Autodesk Inventor part; units mm, degrees
ref_plane "YZ Plane" through (0, 0, 0) normal (1, 0, 0) x (0, 1, 0)
ref_plane "XZ Plane" through (0, 0, 0) normal (0, 1, 0) x (-1, 0, 0)
ref_plane "XY Plane" through (0, 0, 0) normal (0, 0, 1) x (1, 0, 0)
sketch "Skizze1" plane through (0, 0, 0) normal (0, 0, 1) x (1, 0, 0)
  line L0 (0, 0) -> (100, 0)
  line L1 (100, 0) -> (100, 60)
  line L2 (100, 60) -> (0, 60)
  line L3 (0, 60) -> (0, 0)
  dimension "d0" = 100
  dimension "d1" = 60
extrude "Extrusion1" add sketch "Skizze1" along normal blind 12
sketch "Skizze2" plane through (0, 0, 12) normal (0, 0, 1) x (1, 0, 0)
  circle A0 centre (33, 50.3439) radius 3
  circle A1 centre (17, 50.3439) radius 3
  point P0 (0, 0)
  point P1 (25, 45.3439)
hole "Bohrung1" at (17, 50.3439, 12) at (33, 50.3439, 12) direction (0, 0, -1) diameter 6 end through all
sketch "Skizze4" plane through (0, 0, 12) normal (0, 0, 1) x (1, 0, 0)
  circle A0 centre (25, 48.4439) radius 3.1
  point P0 (0, 0)
  point P1 (25, 45.3439)
hole "Bohrung3" at (25, 48.4439, 12) direction (0, 0, -1) diameter 6 end through all
sketch "Skizze6" plane through (0, 0, 0) normal (0, 0, -1) x (-1, 0, 0)
  circle A0 centre (-35, 15) radius 2.5
  point P0 (0, 0)
hole "Bohrung5" at (35, 15, 0) direction (0, 0, 1) diameter 6 end through all
properties part number "Seitenwand"
Geometry: final body of the model. Coordinates: model frame, mm. Give positions to 0.01 mm unless a question says otherwise; leave off trailing zeros. Loops run counter-clockwise (first coordinate to the right, second up) from the corner with the lowest first, then second, coordinate; pieces in that order, holes last. Notation, with made-up numbers: (-7.5, 41.25) - (33.5, 41.25) arc R34 ccw to (33.5, 77.25) - close; hole circle Ø6 at (26.5, -0.5). An arc over 180 degrees is marked (long way). Answer as CSV lines item,"result". Start each with the question number.
(1) Pin query (flat end, axial travel): P1, Ø8, axis at x = 17, y = 50.34, coming from the +Z side. Return the tip coordinate at first contact, or that it passes through.
(2) Section query A-A (x = 17). Output: boundary loops of the cut face in (y, z), and give its area (3 significant figures).
(3) Section query B-B (y = 15). Output: boundary loops of the cut face in (x, z), and give its area (3 significant figures).
(4) Section query C-C (z = 11). Output: boundary loops of the cut face in (x, y).
(5) Section query D-D (x = 33). Output: boundary loops of the cut face in (y, z), and give its area (3 significant figures).
(6) Mould query, pull axis X, two halves, no side actions, for faces 1 (the face through (32.1, 47.48, 5.92)), 2 (the face through (0, 30, 6)), 3 (the face through (49, 30, 12)). Classes: +X half, -X half, draft (parallel to the pull), parting line (faces both ways), or undercut.
(7) Ray query, line 1 along Y through (x, z) = (25, 3.5); line 2 along Y through (x, z) = (35, 4.25); line 3 along X through (y, z) = (14.5, 6). Return the intervals inside material, ascending. Write a range as [from, to].
Worked answers:
1,P1,"stops at z = 12"
2,outline,"(0, 0) - (47.34, 0) - (47.34, 12) - (0, 12) - close; (53.34, 0) - (60, 0) - (60, 12) - (53.34, 12) - close"
2,area,"648 mm^2"
3,outline,"(0, 0) - (32, 0) - (32, 12) - (0, 12) - close; (38, 0) - (100, 0) - (100, 12) - (38, 12) - close"
3,area,"1,130 mm^2"
4,outline,"(0, 0) - (100, 0) - (100, 60) - (0, 60) - close; hole circle Ø6 at (17, 50.34); hole circle Ø6 at (25, 48.44); hole circle Ø6 at (33, 50.34); hole circle Ø6 at (35, 15)"
5,outline,"(0, 0) - (12.76, 0) - (12.76, 12) - (0, 12) - close; (17.24, 0) - (47.34, 0) - (47.34, 12) - (17.24, 12) - close; (53.34, 0) - (60, 0) - (60, 12) - (53.34, 12) - close"
5,area,"594 mm^2"
6,face 1,"undercut"
6,face 2,"-X half"
6,face 3,"draft"
7,line 1,"y = [0, 45.44], [51.44, 60]"
7,line 2,"y = [0, 12], [18, 48.11], [52.58, 60]"
7,line 3,"x = [0, 32.04], [37.96, 100]"
